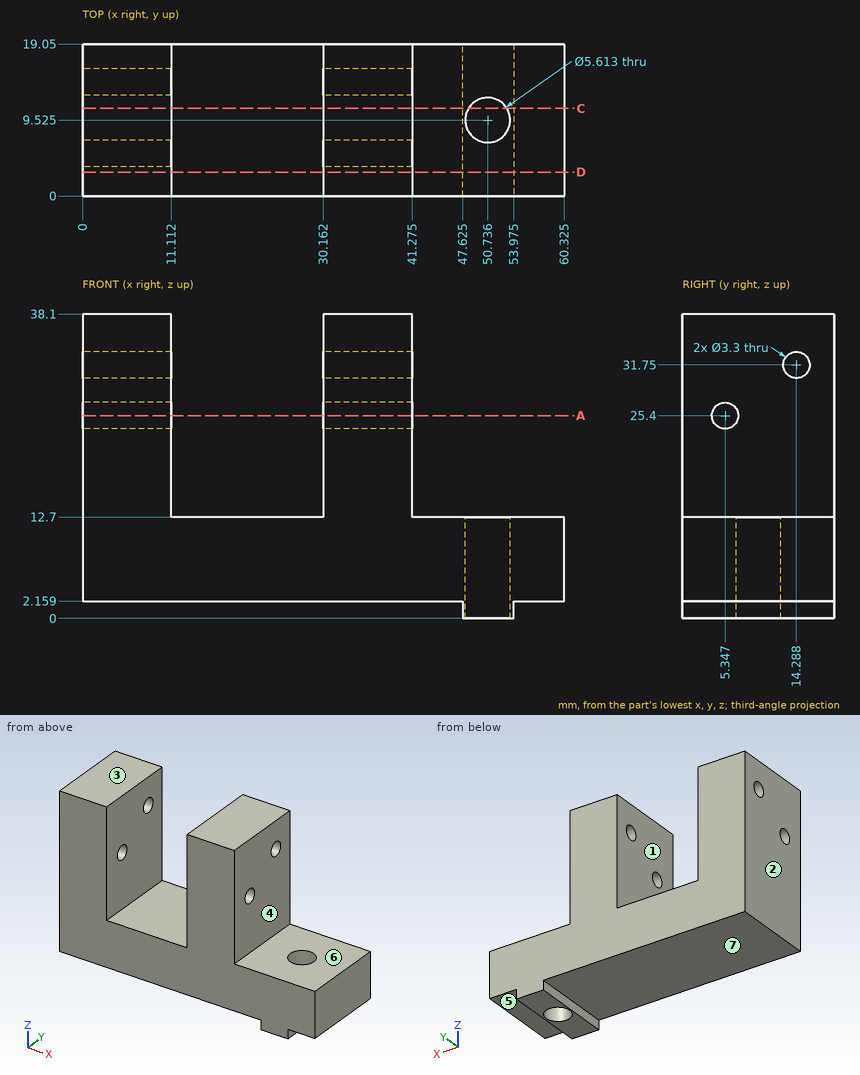
Check sheet for the drawn part. Datum: minimum x, y, z corner. Units: mm. A direction names the side the tool comes from. Give positions to 0.01 mm unless a question says otherwise; leave off trailing zeros. Order: outer loops, then holes, each group sorted by start corner. A loop starts at its lowest first (then second) coordinate and runs counter-clockwise, first axis right, second up. Notation, with made-up numbers: (20, 30) - (32, 30) arc R30 ccw to (32, 59) - close; hole circle Ø11 at (46, 73.5). An arc over 180 degrees is marked (long way). Answer in a Markdown table with one row per item. Add a question column.
Q1. Tool access check on the marked faces 5, 6 and 7. Record the directions out of +Z, -Z, +X, -X, +Y, -Y that give a thin tool (end or side, any length) a straight path to the whole face; none if there is none.
Q2. Material ranges on probe 1 along Y at (x, z) = (2.75, 31.75); probe 2 along X at (y, z) = (6, 14) (1 decimal); probe 3 along Z at (x, y) = (27.5, 7.75), recorded low to high. Write a range as from..to.
Q3. Mould release check, pull along X, two halves, no side actions. Record for the marked faces 1, 2, 3 and 4: pulls with the +X half, pulls with the -X half, needs draft (parallel to the pull), parting line crosses it, or undercut.
Q4. Cross-section at C-C, the plane y = 11. Enter the section's corners in (x, z) (1 decimal), then the cut area to 3 significant figures.
Q5. Gauge pin test, flat ends, axial feed: pin 1 (4.5 mm diameter, centred on y = 5.35, z = 25.4, fed in from +X) (1 decimal); pin 2 (4 mm diameter, centred on x = 47, z = 5.5, fed in from -Y); pin 3 (0.6 mm diameter, centred on y = 13.5, z = 1, fed in from -X) (1 decimal); pin 4 (1.5 mm diameter, centred on x = 49, y = 2.5, fed in from +Z). Record the tip position at first contact, or that the pin passes through.
Q6. Cross-section at A-A, the plane z = 25.4. Count the separate pieces of the cut face and the enclosed holes in it, then the cut area to 3 significant figures.
Q7. Cross-section at D-D, the plane y = 3. Enter the section's corners in (x, z) (1 decimal).
Check values:
| question | item | result |
|---|---|---|
| 1 | face 5 | -Z, +X, +Y, -Y |
| 1 | face 6 | +Z, +X, +Y, -Y |
| 1 | face 7 | -Z, -X, +Y, -Y |
| 2 | probe 1 | y = 0..12.64, 15.94..19.05 |
| 2 | probe 2 | x = 0..11.1, 30.2..41.3 |
| 2 | probe 3 | z = 2.16..12.7 |
| 3 | face 1 | undercut |
| 3 | face 2 | pulls with the -X half |
| 3 | face 3 | needs draft |
| 3 | face 4 | pulls with the +X half |
| 4 | outline | (0, 2.2) - (47.6, 2.2) - (47.6, 0) - (48.3, 0) - (48.3, 12.7) - (41.3, 12.7) - (41.3, 38.1) - (30.2, 38.1) - (30.2, 12.7) - (11.1, 12.7) - (11.1, 38.1) - (0, 38.1) - close; (53.1, 0) - (54, 0) - (54, 2.2) - (60.3, 2.2) - (60.3, 12.7) - (53.1, 12.7) - close |
| 4 | area | 1,150 mm^2 |
| 5 | pin 1 | stops at x = 41.3 |
| 5 | pin 2 | stops at y = 0 |
| 5 | pin 3 | stops at x = 47.6 |
| 5 | pin 4 | stops at z = 12.7 |
| 6 | separate pieces | 4 |
| 6 | enclosed holes | 0 |
| 6 | area | 350 mm^2 |
| 7 | outline | (0, 2.2) - (47.6, 2.2) - (47.6, 0) - (54, 0) - (54, 2.2) - (60.3, 2.2) - (60.3, 12.7) - (41.3, 12.7) - (41.3, 38.1) - (30.2, 38.1) - (30.2, 12.7) - (11.1, 12.7) - (11.1, 38.1) - (0, 38.1) - close |
